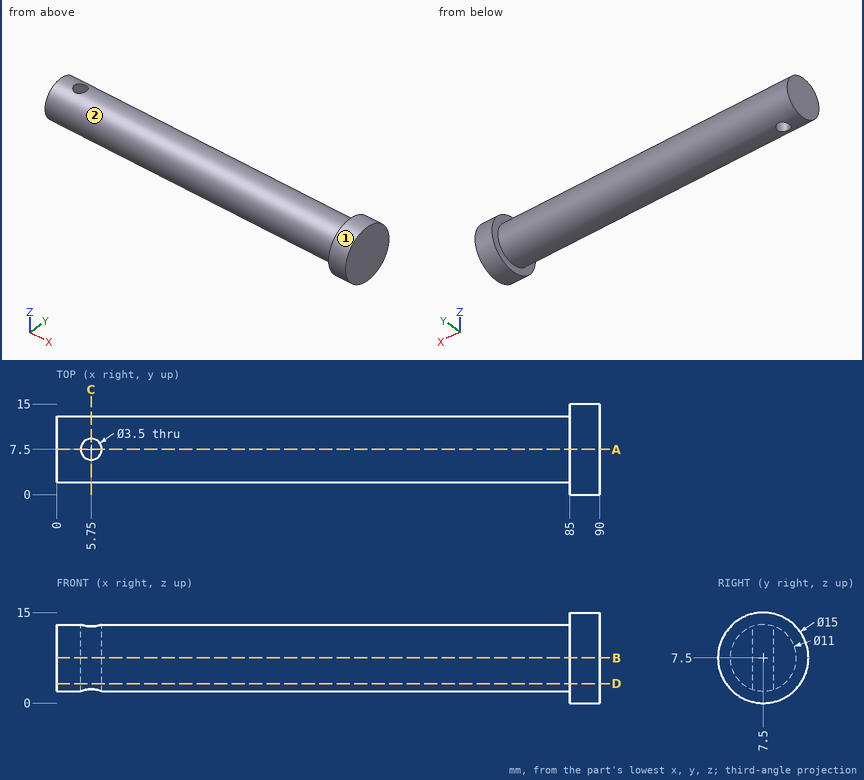
Part print with two shaded views. Sizes in mm from the minimum x, y, z corner. A direction names the side the tool comes from. Round coordinates to 2 decimals unless told otherwise and drop trailing zeros. Loops run counter-clockwise (first coordinate to the right, second up) from the corner with the lowest first, then second, coordinate; pieces in that order, holes last.
Item 1: Saw through at B-B (z = 7.5). List the corners of the cut face in (x, y).
Item 2: Saw through at C-C (x = 5.75). List the corners of the cut face in (y, z).
Item 3: Drill centre lines: line 1 along X through (y, z) = (7.5, 8.75); line 2 along X through (y, z) = (8.5, 13); line 3 along X through (y, z) = (6.25, 7). Where is each one in solid material? Low to high.
Item 4: Which spindle directions (+Z, -Z, +X, -X, +Y, -Y) get a long thin tool onto all of the face, cutting with end or side? Do the marked faces 1 and 2. Say none if no direction does.
Item 5: Pin check, flat tips, straight feed: P1, Ø1.5, axis at x = 38, z = 7, coming from the -Y side; P2, Ø8, axis at x = 48, z = 3.5, coming from the +Y side; P3, Ø5, axis at x = 46.5, y = 10, coming from the +Z side. Stop position of each tip, or through.
Item 6: Saw through at D-D (z = 3.25). List the corners of the cut face in (x, y).
Item 7: Saw through at A-A (y = 7.5). List the corners of the cut face in (x, z), then the cut area to 4 significant figures.
Worked answers:
1. outline: (0, 2) - (85, 2) - (85, 0) - (90, 0) - (90, 15) - (85, 15) - (85, 13) - (0, 13) - close; hole circle Ø3.5 at (5.75, 7.5)
2. outline: (5.75, 2.29) - (5.75, 12.71) arc R5.5 ccw to start; (9.25, 2.29) arc R5.5 ccw to (9.25, 12.71) - close
3. line 1: x = 0 to 4, 7.5 to 90
3. line 2: x = 85 to 90
3. line 3: x = 0 to 4.53, 6.97 to 90
4. face 1: +X, -X
4. face 2: -X
5. P1: stops at y = 2
5. P2: stops at y = 13
5. P3: stops at z = 13
6. outline: (0, 4.01) - (85, 4.01) - (85, 1.32) - (90, 1.32) - (90, 13.68) - (85, 13.68) - (85, 10.99) - (0, 10.99) - close; hole circle Ø3.5 at (5.75, 7.5)
7. outline: (0, 2) - (4, 2) - (4, 13) - (0, 13) - close; (7.5, 2) - (85, 2) - (85, 0) - (90, 0) - (90, 15) - (85, 15) - (85, 13) - (7.5, 13) - close
7. area: 971.5 mm2
